Design review of the part shown in the three views and the two pictorial views. Dimensions are in mm from the part's minimum x, y and z. A direction names the side the tool comes from. Coordinates: 2 decimals unless noted, no trailing zeros. Write each loop counter-clockwise with the first axis right and the second up, starting at its lowest first coordinate (ties: lowest second). Pieces come first, ordered by that corner, then holes. Notation, with made-up numbers: (12, 79.5) - (31, 79.5) arc R21 ccw to (31, 117.5) - close; hole circle Ø11 at (54, -15). An arc over 180 degrees is marked (long way). Write each question's results on one line, items separated by ' | '.
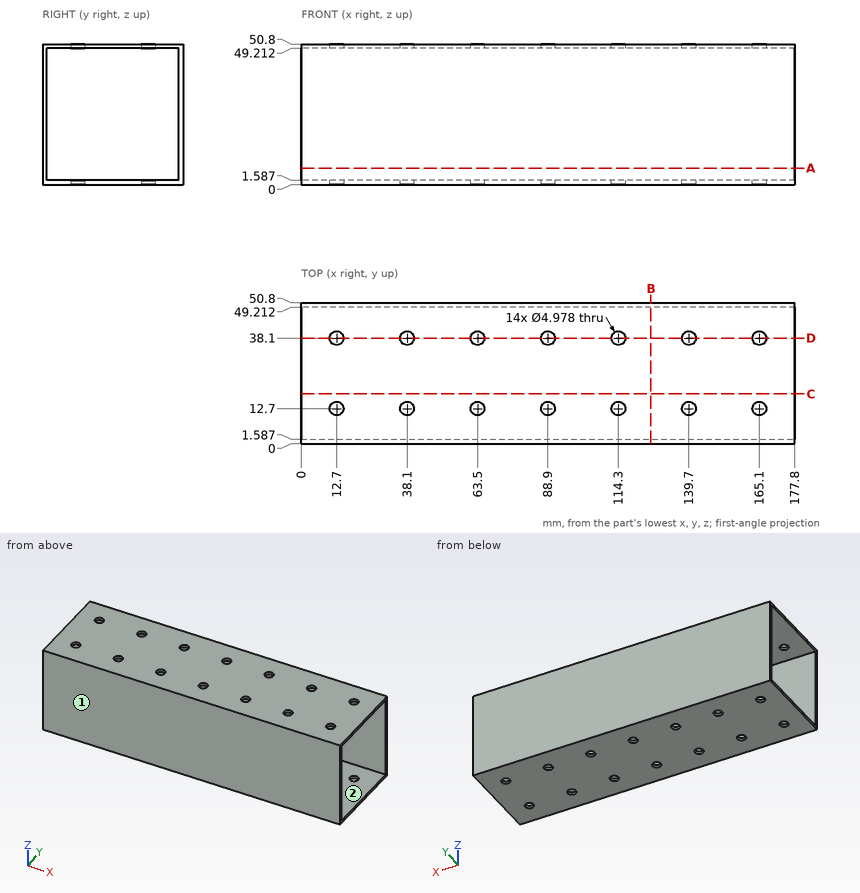
Q1. Take a section at D-D on y = 38.1. State how many separate pieces and enclosed holes the cut face has.
Results found:
separate pieces: 16 | enclosed holes: 0
Q2. For the marked faces 1 and 2, list the 3-axis set-ups (+Z, -Z, +X, -X, +Y, -Y) from which the entire face can be reached by the end or side of a thin tool; tool diameter is ignored.
Results found:
face 1: +Z, -Z, +X, -X, -Y | face 2: +X, -X
Q3. Wall thickness on line 1 along Y through (x, z) = (139.7, 1.2); line 2 along Z through (x, y) = (153, 28): over which ranges is each line inside the solid? List them lowest first. Write a range as from..to.
Results found:
line 1: 0..10.21, 15.19..35.61, 40.59..50.8 | line 2: 0..1.59, 49.21..50.8
Q4. Take a section at B-B on x = 126. State the section outline as (y, z) points.
Results found:
outline: (0, 0) - (50.8, 0) - (50.8, 50.8) - (0, 50.8) - close; hole (1.59, 1.59) - (49.21, 1.59) - (49.21, 49.21) - (1.59, 49.21) - close
Q5. Take a section at A-A on z = 6. State the section outline as (x, y) points.
Results found:
outline: (0, 0) - (177.8, 0) - (177.8, 1.59) - (0, 1.59) - close; (0, 49.21) - (177.8, 49.21) - (177.8, 50.8) - (0, 50.8) - close
